Read the model definition and answer for the solid it produces. Units are mm, in the model's axes. A direction names the side the tool comes from. Round coordinates to 2 decimals unless told otherwise and drop trailing zeros. Order: outer loops, then holes, each group sorted by start corner. A loop starts at its lowest first (then second) coordinate and runs counter-clockwise, first axis right, second up. Notation, with made-up numbers: (33.25, -30) - (78.25, -30) arc R16 ccw to (78.25, -4) - close; hole circle Ø4 at (32.25, 49). An arc over 180 degrees is marked (long way). One line per question, with ' | ' between items. Start each with the question number.
1) The part is cut by section D-D, the plane x = -0.8. Give the vertices of the cut face in (y, z).
2) Flat-ended cylindrical pins translate along their axes: pin 1 (1 mm diameter, centred on y = -27, z = 67, fed in from +X); pin 2 (1.5 mm diameter, centred on x = -0.5, y = -13, fed in from +Z). Find the tip coordinate at first contact, or state that the pin passes through.
3) The mould has two halves that part along Z. Classify faces 1 (the flat face through (-2.46, -12.06, 76.86)), 2 (the flat face through (-5, -16, 71)), 3 (the cylindrical face through (-2.465, -33.966, 73.64)), 4 (the flat face through (-2, -18, 72)): pulls with the +Z half, pulls with the -Z half, needs draft (parallel to the pull), parting line crosses it, or undercut.
4) The part is cut by section B-B, the plane x = -4.35. Give the vertices of the cut face in (y, z), plus the area to 3 significant figures.
5) The part is cut by section C-C, the plane z = 74.25. Give the vertices of the cut face in (x, y), plus the area to 3 significant figures.
6) For faces 5 (the cylindrical face through (-2.46, -0.77, 70.75)), 6 (the cylindrical face through (-0.99, -10.52, 70.95)), determine the directions among +Z, -Z, +X, -X, +Y, -Y from which every point of the face is accessible in a straight line to the end or side of a thin tool.
7) Straight lines are drawn through the part: line 1 (Y direction, x = -2.3, z = 71); line 2 (Y direction, x = -1.15, z = 72); line 3 (Z direction, x = -3.2, y = -1). For each, find the intervals that lie inside material, in ascending order. Write a range as from..to.
Solid Edge part; units mm, degrees
sketch "Sketch1" plane through (0, 0, 0) normal (1, 0, 0) x (0, 1, 0)
  circle A0 centre (-26.5278, 72.6775) radius 3.6
  line L0 (-0.5498, 65.9584) -> (-26.3014, 65.1809)
  line L1 (0.2798, 73.842) -> (-24.746, 79.9627)
  arc A1 (0.2798, 73.842) -> (-0.5498, 65.9583) centre (-0.6705, 69.9565) cw
  arc A2 (-26.3014, 65.1809) -> (-24.746, 79.9628) centre (-26.5278, 72.6775) cw
  circle A3 centre (-0.6705, 69.9565) radius 0.8
extrude "Protrusion1" add sketch "Sketch1" against normal blind 5
sketch "Sketch2" plane through (0, -15.3492, 72.6775) normal (1, 0, 0) x (0, 0.9995, 0.0302)
  circle A0 centre (1.2127, -1.3453) radius 0.8
extrude "Cutout1" cut sketch "Sketch2" against normal up to next
sketch "Sketch3" plane through (0, -15.3492, 72.6775) normal (1, 0, 0) x (0, 0.9995, 0.0302)
  line L0 (-10.3095, 3.8321) -> (3.2031, 0.4913)
  arc A0 (3.2031, 0.4913) -> (2.6407, -3.6465) centre (2.699, -1.5473) cw
  line L1 (2.6407, -3.6465) -> (-11.1721, -3.2627)
  arc A1 (-11.1721, -3.2627) -> (-10.3095, 3.8321) centre (-11.1735, 0.3373) cw
extrude "Cutout2" cut sketch "Sketch3" against normal blind 2
Values:
1) outline: (-26.3, 65.18) - (-0.55, 65.96) arc R4 ccw to (0.28, 73.84) - (-24.75, 79.96) arc R7.5 ccw (long way) to start; hole (-30.13, 72.56) arc R3.6 ccw to (-26.42, 69.08) - (-12.6, 69.11) arc R2.1 ccw to (-12.16, 73.27) - (-25.72, 76.19) arc R3.6 ccw to start; hole circle Ø1.6 at (-0.67, 69.96)
2) pin 1: stops at x = 0 | pin 2: stops at z = 77.27
3) face 1: pulls with the +Z half | face 2: needs draft | face 3: parting line crosses it | face 4: undercut
4) outline: (-26.3, 65.18) - (-0.55, 65.96) arc R4 ccw to (0.28, 73.84) - (-24.75, 79.96) arc R7.5 ccw (long way) to start; hole circle Ø7.2 at (-26.53, 72.68); hole circle Ø1.6 at (-14.1, 71.37); hole circle Ø1.6 at (-0.67, 69.96) | area: 370 mm^2
5) outline: (-5, -33.86) - (0, -33.86) - (0, -29.77) - (-5, -29.77) - close; (-5, -23.29) - (-2, -23.29) - (-2, -16.73) - (0, -16.73) - (0, -1.39) - (-5, -1.39) - close | area: 117 mm^2
6) face 5: +X, -X | face 6: +X
7) line 1: y = -33.84..-29.71, -23.34..-14.81, -13.39..3.19 | line 2: y = -34..-30.06, -10.66..2.77 | line 3: z = 65.94..69.23, 70.69..74.15
